```python
from build123d import *

# Parameters (mm, degrees)
SKETCH1_W                = 38.1
SKETCH1_H                = 38.1
SKETCH1_R                = 11.43
BOSS_EXTRUDE1_DEPTH      = 3.175
SKETCH2_R                = 1.6002
SKETCH2_R_2              = 1.4351
CUT_EXTRUDE1_DEPTH       = 28.127211891
CIRPATTERN1_COUNT        = 4
CHAMFER1_SIZE            = 2.54
BOSS_EXTRUDE2_START      = 3.175
SKETCH3_R                = 1.4351
BOSS_EXTRUDE2_DEPTH      = 3.175
FILLET1_R                = 1.905
CIRPATTERN7_COUNT        = 4
FILLET1_OF_CIRPATTERN7_R = 1.905


with BuildPart() as part:
    # Sketch1 → Boss-Extrude1 (new body)
    with BuildSketch(Plane(origin=(0, 0, 0), x_dir=(1, 0, 0), z_dir=(0, 1, 0))):
        Rectangle(SKETCH1_W, SKETCH1_H)
        with Locations(Location((0, 0, 0), (0, 0, 270))):
            Circle(SKETCH1_R, mode=Mode.SUBTRACT)
    extrude(amount=BOSS_EXTRUDE1_DEPTH)

    # Sketch2 → Cut-Extrude1 (cut, through all)
    with BuildSketch(Plane(origin=(0, 3.175, 0), x_dir=(1, 0, 0), z_dir=(0, 1, 0))):
        with Locations(Location((0, 13.9954, 0), (0, 0, 270))):
            Circle(SKETCH2_R)
        with Locations(Location((15.24, 15.24, 0), (0, 0, 270))):
            Circle(SKETCH2_R_2)
    cut_extrude1 = extrude(amount=-CUT_EXTRUDE1_DEPTH, mode=Mode.SUBTRACT)

    # CirPattern1: Cut-Extrude1 ×4 about axis
    cirpattern1_axis = Axis((0, 0, 0), (0, 1, 0))
    for i in range(1, CIRPATTERN1_COUNT):
        add(cut_extrude1.rotate(cirpattern1_axis, i * 360 / CIRPATTERN1_COUNT), mode=Mode.SUBTRACT)

    # Chamfer1
    chamfer1_edges = [part.edges().sort_by_distance(p)[0] for p in [
        (19.05, 1.5875, 19.05),
        (-19.05, 1.5875, 19.05),
        (-19.05, 1.5875, -19.05),
        (19.05, 1.5875, -19.05),
    ]]
    chamfer(chamfer1_edges, length=CHAMFER1_SIZE)

    # Sketch3 → Boss-Extrude2 (add)
    with BuildSketch(Plane(origin=(0, 3.175, 0), x_dir=(1, 0, 0), z_dir=(0, 1, 0)).offset(BOSS_EXTRUDE2_START)):
        with BuildLine():
            Line((-19.05, 16.51), (-19.05, 11.43))
            Line((-19.05, 11.43), (-14.438397591, 11.43))
            ThreePointArc((-14.438397591, 11.43), (-13.021371376, 13.021371376), (-11.43, 14.438397591))
            Line((-11.43, 14.438397591), (-11.43, 19.05))
            Line((-11.43, 19.05), (-16.51, 19.05))
            Line((-16.51, 19.05), (-19.05, 16.51))
        make_face()
        with Locations((-15.24, 15.24)):
            Circle(SKETCH3_R, mode=Mode.SUBTRACT)
    boss_extrude2 = extrude(amount=-BOSS_EXTRUDE2_DEPTH)

    # Fillet1
    fillet1_edges = [part.edges().sort_by_distance(p)[0] for p in [
        (-11.43, 4.7625, -19.05),
        (-19.05, 4.7625, -11.43),
        (-14.438397591, 4.7625, -11.43),
        (-11.43, 4.7625, -14.438397591),
    ]]
    fillet(fillet1_edges, radius=FILLET1_R)

    # CirPattern7: Boss-Extrude2 ×4 about axis
    cirpattern7_axis = Axis((0, 0, 0), (0, 1, 0))
    for i in range(1, CIRPATTERN7_COUNT):
        add(boss_extrude2.rotate(cirpattern7_axis, i * 360 / CIRPATTERN7_COUNT))

    # Fillet1 of CirPattern7
    fillet1_of_cirpattern7_edges = [part.edges().sort_by_distance(p)[0] for p in [
        (-19.05, 4.7625, 11.43),
        (-11.43, 4.7625, 19.05),
        (-11.43, 4.7625, 14.438397591),
        (-14.438397591, 4.7625, 11.43),
        (11.43, 4.7625, 19.05),
        (19.05, 4.7625, 11.43),
        (14.438397591, 4.7625, 11.43),
        (11.43, 4.7625, 14.438397591),
        (19.05, 4.7625, -11.43),
        (11.43, 4.7625, -19.05),
        (11.43, 4.7625, -14.438397591),
        (14.438397591, 4.7625, -11.43),
    ]]
    fillet(fillet1_of_cirpattern7_edges, radius=FILLET1_OF_CIRPATTERN7_R)


solid = part.part
```
CAD build for the part. Positions are in the model's coordinates, mm. A direction names the side the tool comes from. Coordinates: 2 decimals unless noted, no trailing zeros. Order: outer loops, then holes, each group sorted by start corner. A loop starts at its lowest first (then second) coordinate and runs counter-clockwise, first axis right, second up. Notation, with made-up numbers: M 61,72.5 L 92,72.5 A25 cw 92,108.5 Z; hole C 48.5,-26.75 d10. An arc over 180 degrees is marked long. Write each question's results on one line, items separated by ' | '. Start each with the question number.
Q1. Pull direction Z, two halves, no side cores. Call faces 1 (the flat face through (17.8, 3.22, -17.76)), 2 (the flat face through (17.76, 3.22, 17.8)), 3 (the flat face through (-11.43, 5, -16)), 4 (the cylindrical face through (11.333, 1.565, -1.488)): +Z half, -Z half, draft (parallel to the pull), parting line (faces both ways), or undercut.
Q2. Cut at A-A (y = 1.5). Count the separate pieces of the cut face and the enclosed holes in it, then the cut area to 3 significant figures.
Q3. Cut at D-D (z = 8). List the corners of the cut face in (x, y) (3 decimals).
Q4. Cut at C-C (x = -3.5). List the corners of the cut face in (y, z) (3 decimals).
Q5. Flat gauge pins, fed straight in: P1, Ø4, axis at x = 0, z = -14, coming from the -Y side; P2, Ø2.5, axis at x = 15.24, z = 15.24, coming from the -Y side; P3, Ø11.5, axis at x = -6, z = -5.5, coming from the +Y side (3 decimals). Where does each tip first touch, or does it go through?
Q6. Cut at B-B (z = 0). List the corners of the cut face in (x, y) (3 decimals), then the cut area to 3 significant figures.
Q7. Drill centre lines: probe 1 along Z at (x, y) = (-15.24, 4); probe 2 along X at (y, z) = (2.5, 1); probe 3 along X at (y, z) = (1.5, -15.24). Where is each one in solid material? Low to high. Write a range as from..to.
Q8. Which spindle directions (+Z, -Z, +X, -X, +Y, -Y) get a long thin tool onto all of the face, cutting with end or side? Do faces 5 (the flat face through (16, 5, -11.43)), 6 (the cylindrical face through (18.477, 4.74, -11.973)), 7 (the cylindrical face through (-14.55, 4.74, 11.6)), 8 (the flat face through (-11.43, 5, 16)). Say none if no direction does.
Found:
1) face 1: -Z half | face 2: +Z half | face 3: draft | face 4: undercut
2) separate pieces: 1 | enclosed holes: 9 | area: 970 mm²
3) outline: M -19.05,0 L -8.164,0 L -8.164,3.175 L -19.05,3.175 Z; M 8.164,0 L 19.05,0 L 19.05,3.175 L 8.164,3.175 Z
4) outline: M 0,-19.05 L 3.175,-19.05 L 3.175,-10.881 L 0,-10.881 Z; M 0,10.881 L 3.175,10.881 L 3.175,19.05 L 0,19.05 Z
5) P1: y = 0 | P2: through | P3: y = 3.175
6) outline: M -19.05,0 L -15.596,0 L -15.596,3.175 L -19.05,3.175 Z; M -12.395,0 L -11.43,0 L -11.43,3.175 L -12.395,3.175 Z; M 11.43,0 L 12.395,0 L 12.395,3.175 L 11.43,3.175 Z; M 15.596,0 L 19.05,0 L 19.05,3.175 L 15.596,3.175 Z | area: 28.1 mm²
7) probe 1: -19.05..-16.68, -13.8..-11.43, 11.43..13.8, 16.68..19.05 | probe 2: -19.05..-15.24, -12.75..-11.39, 11.39..12.75, 15.24..19.05 | probe 3: -19.05..-16.68, -13.8..-1.01, 1.01..13.8, 16.68..19.05
8) face 5: +X, -X, +Y | face 6: +X, +Y | face 7: +Y | face 8: +Z, -Z, +Y
